Geometry check sheet. Reference: the model listing, model coordinates, mm. Give positions to 0.01 mm unless a question says otherwise; leave off trailing zeros. Order: outer loops, then holes, each group sorted by start corner. A loop starts at its lowest first (then second) coordinate and runs counter-clockwise, first axis right, second up. Notation, with made-up numbers: M -10,-25 L 46,-25 A20 cw 46,-8 Z; hole C 43,-39 d1. An arc over 180 degrees is marked long. Put each result on its own line as item: value. Start each with the question number.
Q1. Go/stop test with flat-tipped pins: pin 1 (6 mm diameter, centred on x = 3.5, y = -18, fed in from -Z); pin 2 (5 mm diameter, centred on y = 135, z = -3, fed in from +X); pin 3 (1 mm diameter, centred on y = -127.5, z = 3, fed in from +X). Record where each tip stops, or that it passes through.
Q2. Material ranges on L1, parallel to X at y = 89, z = 0; L2, parallel to Y at x = 3, z = 0; L3, parallel to X at y = -55, z = 1.5, recorded low to high.
Q3. Section check B-B on y = 39.5. Record the cut outline in (x, z), then the cut area to 3 significant figures.
Q4. Section check A-A on z = 0. Record the cut outline in (x, y).
```python
from build123d import *

# Parameters (mm, degrees)
SKETCH1_R               = 5.5
BOSS_EXTRUDE2_DEPTH     = 177.8
SKETCH4_R               = 2.5
CUT_EXTRUDE1_DEPTH      = 356.685057319
CUT_EXTRUDE3_REACH      = 180.559
CUT_EXTRUDE3_END_RADIUS = 2.5
SKETCH7_R               = 2.5


with BuildPart() as part:
    # Sketch1 → Boss-Extrude2 (new, symmetric)
    with BuildSketch(Plane(origin=(0, 0, 0), x_dir=(1, 0, 0), z_dir=(0, 1, 0))):
        with Locations(Location((0, 0, 0), (0, 0, 270))):
            Circle(SKETCH1_R)
    extrude(amount=BOSS_EXTRUDE2_DEPTH, both=True)

    # Sketch4 → Cut-Extrude1 (cut, through all)
    with BuildSketch(Plane(origin=(0, 177.8, 0), x_dir=(1, 0, 0), z_dir=(0, 1, 0))):
        with Locations(Location((0, 0, 0), (0, 0, 270))):
            Circle(SKETCH4_R)
    extrude(amount=-CUT_EXTRUDE1_DEPTH, mode=Mode.SUBTRACT)

    # Cut-Extrude3: up to this cylinder (the profile starts outside it)
    cut_extrude3_end = Plane(origin=(0, -128.8, 0), z_dir=(0, 1, 0)) * Cylinder(CUT_EXTRUDE3_END_RADIUS, 367.118, mode=Mode.PRIVATE)
    # Sketch7 → Cut-Extrude3 (cut, up to the surface)
    with BuildSketch(Plane(origin=(10, 0, 0), x_dir=(0, 0, -1), z_dir=(1, 0, 0)), mode=Mode.PRIVATE) as cut_extrude3_sk1:
        with Locations((0, -128.8)):
            Circle(SKETCH7_R)
    cut_extrude3_tool1 = extrude(cut_extrude3_sk1.sketch, amount=-CUT_EXTRUDE3_REACH, mode=Mode.PRIVATE) - cut_extrude3_end
    add(cut_extrude3_tool1.solids().sort_by_distance((10, -128.8, 0))[0], mode=Mode.SUBTRACT)


solid = part.part
```
Results found:
1. pin 1: stops at z = -5.48
1. pin 2: stops at x = 5.48
1. pin 3: stops at x = 4.9
2. L1: x = -5.5 to -2.5, 2.5 to 5.5
2. L2: y = -177.8 to -131.3, -126.3 to 177.8
2. L3: x = -5.29 to -2, 2 to 5.29
3. outline: C 0,0 d11; hole C 0,0 d5
3. area: 75.4 mm^2
4. outline: M -5.5,-177.8 L -2.5,-177.8 L -2.5,177.8 L -5.5,177.8 Z; M 2.5,-177.8 L 5.5,-177.8 L 5.5,-131.3 L 2.5,-131.3 Z; M 2.5,-126.3 L 5.5,-126.3 L 5.5,177.8 L 2.5,177.8 Z
